Autodesk Inventor part; units mm, degrees
ref_plane "YZ Plane" through (0, 0, 0) normal (1, 0, 0) x (0, 1, 0)
ref_plane "XZ Plane" through (0, 0, 0) normal (0, 1, 0) x (-1, 0, 0)
ref_plane "XY Plane" through (0, 0, 0) normal (0, 0, 1) x (1, 0, 0)
sketch "Boceto1" plane through (0, 0, 0) normal (0, 1, 0) x (-1, 0, 0)
  line L0 (-28.5, 6.5) -> (28.5, 6.5)
  line L1 (28.5, 6.5) -> (28.5, -6.5)
  line L2 (28.5, -6.5) -> (-28.5, -6.5)
  line L3 (-28.5, -6.5) -> (-28.5, 6.5)
  line L4 (-28.5, 6.5) -> (28.5, -6.5) construction
  line L5 (28.5, 6.5) -> (-28.5, -6.5) construction
  line L6 (82.5, 9.5) -> (28.5, 9.5)
  line L7 (28.5, 9.5) -> (28.5, -9.5)
  line L8 (28.5, -9.5) -> (82.5, -9.5)
  line L9 (82.5, -9.5) -> (82.5, 9.5)
  line L10 (-28.5, 9.5) -> (-82.5, 9.5)
  line L11 (-82.5, 9.5) -> (-82.5, -9.5)
  line L12 (-82.5, -9.5) -> (-28.5, -9.5)
  line L13 (-28.5, -9.5) -> (-28.5, 9.5)
  point P0 (0, 0)
  point P1 (28.5, 6.5)
  point P2 (-28.5, 6.5)
  point P3 (28.5, -6.5)
  dimension "d0" = 13
  dimension "d1" = 57
  dimension "d2" = 19
  dimension "d3" = 9.5
  dimension "d4" = 9.5
  dimension "d5" = 19
  dimension "d6" = 165
extrude "Extrusión1" add sketch "Boceto1" along normal mid plane 6
sketch "Boceto3" plane through (0, 3, 0) normal (0, 1, 0) x (1, 0, 0)
  circle A0 centre (-28.5074, -44.5) radius 38
  line L0 (-28.5, -6.5) -> (28.5, -6.5)
  circle A1 centre (-28.5074, 44.5) radius 38
  circle A2 centre (29.8049, 44.5) radius 38
  circle A3 centre (29.8049, -44.5) radius 38
  line L1 (28.5, 6.5) -> (-28.5, 6.5)
  point P0 (0, 0)
  point P1 (0.6488, -68.8704)
  point P2 (0.6488, -20.1296)
  point P3 (0.6488, 68.8704)
  point P4 (0.6488, 20.1296)
  dimension "d11" = 76
extrude "Extrusión2" cut sketch "Boceto3" against normal through all
properties part number "TensileTestSpecimen"
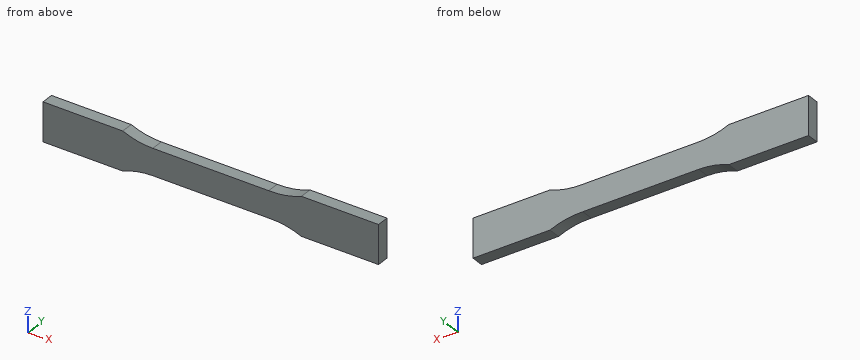
Can you work these out from the model? Positions are in its coordinate system, mm. Coordinates: 2 decimals unless noted, no trailing zeros. Order: outer loops, then holes, each group sorted by start corner. A loop starts at its lowest first (then second) coordinate and runs counter-clockwise, first axis right, second up.
1. If we section it at B-B (z = -8): Please give me the cut outline in (x, y), then the cut area to 3 significant figures.
2. I need wall thicknesses on line 1 (Z direction, x = 26, y = -1.9); line 2 (Z direction, x = 39, y = -1.7). Which ranges of each line are inside material? Lowest first, please.
3. I'm going to push flat-ended pins straight in: pin 1 (2 mm diameter, centred on x = -5, y = 0, fed in from -Z); pin 2 (2 mm diameter, centred on x = -32.5, y = 0, fed in from -Z). Where does each tip first touch, or does it pass through?
4. If we section it at C-C (x = -22.5): Please give me the cut outline in (y, z).
Entries:
1. outline: (-82.5, -3) - (-39.08, -3) - (-39.08, 3) - (-82.5, 3) - close; (40.38, -3) - (82.5, -3) - (82.5, 3) - (40.38, 3) - close
1. area: 513 mm2
2. line 1: z = -6.5 to 6.5
2. line 2: z = -7.63 to 7.63
3. pin 1: stops at z = -6.5
3. pin 2: stops at z = -6.83
4. outline: (-3, -6.5) - (3, -6.5) - (3, 6.5) - (-3, 6.5) - close
